Solid Edge part; units mm, degrees
sketch "Sketch1" plane through (0, 0, 0) normal (1, 0, 0) x (0, 1, 0)
  line L0 (-7.5, 15) -> (-7.5, 0)
  line L1 (-7.5, 0) -> (7.5, 0)
  line L2 (7.5, 0) -> (7.5, 15)
  line L3 (7.5, 15) -> (6, 15)
  line L4 (6, 15) -> (6, 5)
  line L5 (6, 5) -> (-6, 5)
  line L6 (-6, 5) -> (-6, 15)
  line L7 (-6, 15) -> (-7.5, 15)
  dimension "D1" = 7.5
  dimension "D2" = 6
  dimension "D3" = 7.5
  dimension "D4" = 6
extrude "Protrusion1" add sketch "Sketch1" along normal mid plane 12
hole "hole" at (0, 0, 0) direction (0, 0, 1) diameter 2.75 depth 30 tip angle 118 start chamfer 0.6 start chamfer angle 30 end chamfer 0.6 end chamfer angle 30
sketch "Sketch2" plane through (6, 0, 7.5) normal (1, 0, 0) x (0, 0, 1)
  line L0 (-7.5, 7.5) -> (7.5, 7.5)
  line L1 (7.5, 7.5) -> (7.5, -7.5)
  line L2 (7.5, -7.5) -> (-7.5, -7.5)
  line L3 (-7.5, -7.5) -> (-7.5, 7.5)
extrude "wall" add sketch "Sketch2" along normal blind 2
sketch "Sketch3" plane through (8, 0, 7.5) normal (1, 0, 0) x (0, -1, 0)
  line L0 (-3.75, -7.5) -> (3.75, -7.5)
  line L1 (3.75, 2.5) -> (3.75, -7.5)
  line L2 (-3.75, 2.5) -> (3.75, 2.5)
  line L3 (-3.75, -7.5) -> (-3.75, 2.5)
  dimension "D1" = 3.75
  dimension "D2" = 3.75
extrude "Cutout1" cut sketch "Sketch3" against normal up to next
properties material "Polyethylene, low density"
Work out the finished part from the listing and answer in its coordinate system (mm). A direction names the side the tool comes from. Round coordinates to 2 decimals unless told otherwise and drop trailing zeros. Loops run counter-clockwise (first coordinate to the right, second up) from the corner with the lowest first, then second, coordinate; pieces in that order, holes last. Notation, with made-up numbers: M 63.25,38.25 L 117.25,38.25 A25 ccw 117.25,53.25 Z; hole C 70,63 d2. An arc over 180 degrees is marked long. One line per question, with ' | ' between items. Start each with the question number.
(1) For a pull along Y with two mould halves and no side action, classify faces 1 (the face through (0, 6, 10)), 2 (the face through (0.9, -6.5, 15)), 3 (the face through (1, -7.5, 8)) as released by +Y, released by -Y, zero draft, split by the parting line, or undercut.
(2) A cutting plane is placed at B-B on z = 7.25. Write down the section's boundary in (x, y), plus the area to 3 significant figures.
(3) A cutting plane is placed at C-C on x = 0. Write down the section's boundary in (y, z) (3 decimals).
(4) A cutting plane is placed at A-A on y = 0. Write down the section's boundary in (x, z) (3 decimals).
(5) Flat-ended cylindrical pins translate along their axes: pin 1 Ø2.5 at (y, z) = (4.5, 10.5) entering from -X; pin 2 Ø3.5 at (x, y) = (0, 0) entering from -Z; pin 3 Ø1.5 at (x, y) = (-3.5, 2) entering from +Z. Find the tip coordinate at first contact, or state that the pin passes through.
(6) A cutting plane is placed at D-D on z = 3. Write down the section's boundary in (x, y) (3 decimals).
(7) A tool of negligible diameter and unlimited length cuts with its end or side. For faces 4 (the face through (1, 7.5, 7)), 5 (the face through (7, -3.75, 10)), 6 (the face through (6, 5, 10)), from which of +Z, -Z, +X, -X, +Y, -Y can it reach the whole face along a straight path? Write none if from no direction.
(8) Find the intervals of material crossed by line 1 (Y direction, x = 5.75, z = 9.25); line 2 (Y direction, x = 0, z = 1.65) (3 decimals); line 3 (X direction, y = 0, z = 2.4) (3 decimals), in increasing order.
Geometry check:
1) face 1: undercut | face 2: zero draft | face 3: released by -Y
2) outline: M -6,-7.5 L 8,-7.5 L 8,-3.75 L 6,-3.75 L 6,-6 L -6,-6 Z; M -6,6 L 6,6 L 6,3.75 L 8,3.75 L 8,7.5 L -6,7.5 Z | area: 51.0 mm²
3) outline: M -7.5,0 L -1.975,0 L -1.375,1.039 L -1.375,3.961 L -1.975,5 L -6,5 L -6,15 L -7.5,15 Z; M 1.375,1.039 L 1.975,0 L 7.5,0 L 7.5,15 L 6,15 L 6,5 L 1.975,5 L 1.375,3.961 Z
4) outline: M -6,0 L -1.975,0 L -1.375,1.039 L -1.375,3.961 L -1.975,5 L -6,5 Z; M 1.375,1.039 L 1.975,0 L 8,0 L 8,5 L 1.975,5 L 1.375,3.961 Z
5) pin 1: stops at x = 6 | pin 2: stops at z = 0.39 | pin 3: stops at z = 5
6) outline: M -6,-7.5 L 8,-7.5 L 8,7.5 L -6,7.5 Z; hole C 0,0 d2.75
7) face 4: +Z, -Z, +X, -X, +Y | face 5: +Z, +X, -X | face 6: +Z, -X
8) line 1: y = -7.5 to -6, 6 to 7.5 | line 2: y = -7.5 to -1.375, 1.375 to 7.5 | line 3: x = -6 to -1.375, 1.375 to 8
